Job drawing, mm, ordinate dimensions from the low corner. One solid piece. A direction names the side the tool comes from. Give positions to 0.01 mm unless a question says otherwise; leave off trailing zeros. Order: outer loops, then holes, each group sorted by start corner. A loop starts at its lowest first (then second) coordinate and runs counter-clockwise, first axis right, second up. Notation, with made-up numbers: (69.25, -24) - (78.25, -24) arc R13 ccw to (78.25, -15) - close; hole circle Ø1 at (50, -21). An arc over 180 degrees is marked (long way). One line per item, written item: value.
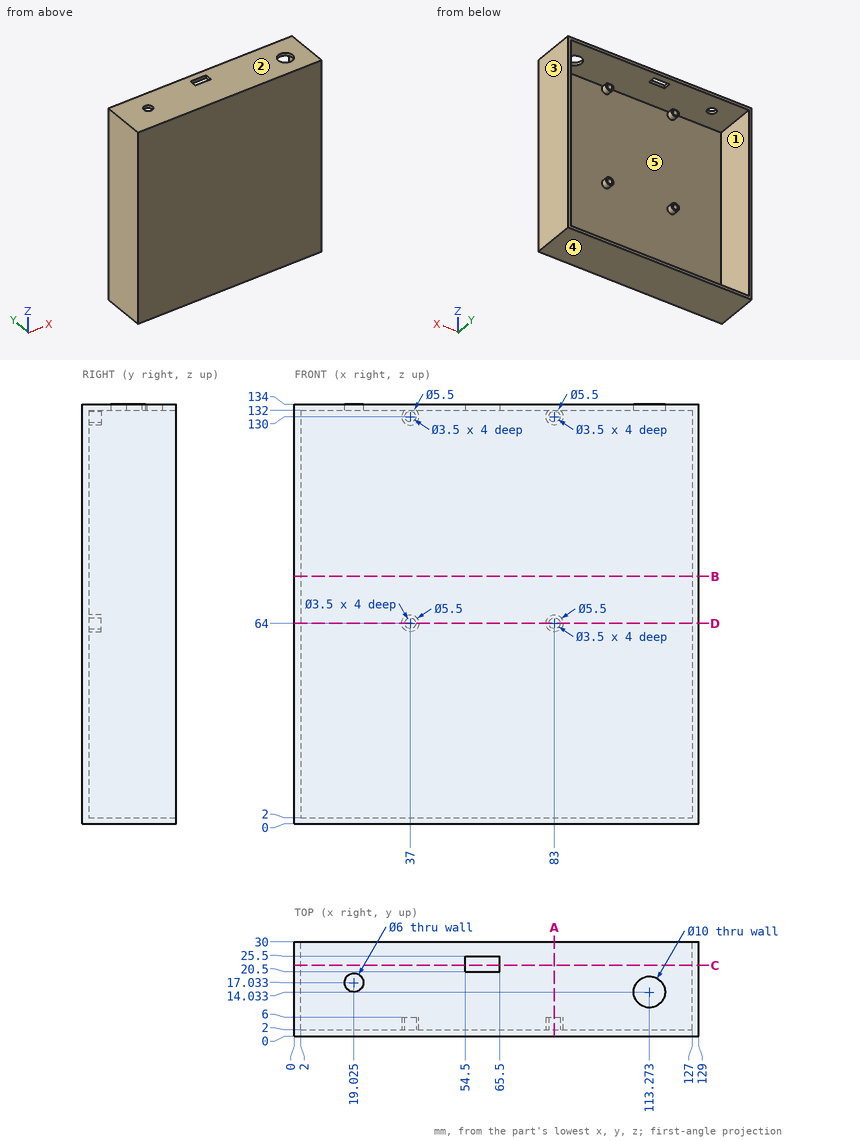
1) Drop flat-ended pins along their axis: P1, Ø1, axis at x = 83.5, z = 64, coming from the +Y side; P2, Ø4, axis at x = 39, z = 117.5, coming from the -Y side; P3, Ø4.5, axis at x = 35.5, z = 63, coming from the +Y side; P4, Ø6, axis at x = 113.27, y = 14.03, coming from the +Z side. Give the stop position or say it passes through.
Answer:
P1: stops at y = 2
P2: stops at y = 0
P3: stops at y = 6
P4: stops at z = 2
2) Slice it at C-C on y = 22.5. Write the cut outline in (x, z).
Answer:
outline: (0, 0) - (129, 0) - (129, 134) - (65.5, 134) - (65.5, 132) - (127, 132) - (127, 2) - (2, 2) - (2, 132) - (54.5, 132) - (54.5, 134) - (0, 134) - close
3) Slice it at A-A on x = 83. Write the cut outline in (y, z).
Answer:
outline: (0, 0) - (30, 0) - (30, 2) - (2, 2) - (2, 61.25) - (6, 61.25) - (6, 62.25) - (2, 62.25) - (2, 65.75) - (6, 65.75) - (6, 66.75) - (2, 66.75) - (2, 127.25) - (6, 127.25) - (6, 128.25) - (2, 128.25) - (2, 131.75) - (6, 131.75) - (6, 132) - (30, 132) - (30, 134) - (0, 134) - close
4) Which spindle directions (+Z, -Z, +X, -X, +Y, -Y) get a long thin tool onto all of the face, cutting with end or side? Do the marked faces 4 and 5. Say none if no direction does.
Answer:
face 4: -Z, +X, -X, +Y, -Y
face 5: +Y
5) Slice it at B-B on z = 79. Write the cut outline in (x, y), then the cut area to 3 significant figures.
Answer:
outline: (0, 0) - (129, 0) - (129, 30) - (127, 30) - (127, 2) - (2, 2) - (2, 30) - (0, 30) - close
area: 370 mm2
6) Wall check: line 1 along Z through (x, y) = (83, 4.2); line 2 along X through (y, z) = (5.2, 130); line 3 along Z through (x, y) = (87, 16). Give the ranges that are in metal, low to high. Write a range as [from, to].
Answer:
line 1: z = [0, 2], [61.25, 62.25], [65.75, 66.75], [127.25, 128.25], [131.75, 134]
line 2: x = [0, 2], [34.25, 35.25], [38.75, 39.75], [80.25, 81.25], [84.75, 85.75], [127, 129]
line 3: z = [0, 2], [132, 134]
7) Slice it at D-D on z = 64. Write the cut outline in (x, y), then the cut area to 3 significant figures.
Answer:
outline: (0, 0) - (129, 0) - (129, 30) - (127, 30) - (127, 2) - (85.75, 2) - (85.75, 6) - (84.75, 6) - (84.75, 2) - (81.25, 2) - (81.25, 6) - (80.25, 6) - (80.25, 2) - (39.75, 2) - (39.75, 6) - (38.75, 6) - (38.75, 2) - (35.25, 2) - (35.25, 6) - (34.25, 6) - (34.25, 2) - (2, 2) - (2, 30) - (0, 30) - close
area: 386 mm2
8) Two-plate mould, pull along Z, no slides. Class the marked faces 1, 2 and 3: pulls with the +Z half, pulls with the -Z half, needs draft (parallel to the pull), parting line crosses it, or undercut.
Answer:
face 1: undercut
face 2: pulls with the +Z half
face 3: needs draft
